```python
from build123d import *

# Parameters (mm, degrees)
BOSS_EXTRUDE1_DEPTH = 44
FILLET1_R           = 10
SKETCH5_W           = 3
SKETCH5_H           = 24
BOSS_EXTRUDE3_DEPTH = 15
FILLET4_R           = 1
CHAMFER3_SIZE       = 1


with BuildPart() as part:
    # Sketch1 → Boss-Extrude1 (new body)
    with BuildSketch(Plane.XY):
        Polygon((-20.6, 0), (20.6, 0), (20.6, 8.604532937), (-20.6, 5), align=None)
    extrude(amount=BOSS_EXTRUDE1_DEPTH)

    # Fillet1
    fillet1_edges = [part.edges().sort_by_distance(p)[0] for p in [
        (20.6, 4.302266469, 44),
        (-20.6, 2.5, 44),
        (20.6, 4.302266469, 0),
        (-20.6, 2.5, 0),
    ]]
    fillet(fillet1_edges, radius=FILLET1_R)

    # Sketch5 → Boss-Extrude3 (add)
    with BuildSketch(Plane.XZ):
        with Locations((19.1, 22)):
            Rectangle(SKETCH5_W, SKETCH5_H)
    extrude(amount=BOSS_EXTRUDE3_DEPTH)

    # Fillet4
    fillet4_edges = [part.edges().sort_by_distance(p)[0] for p in [
        (17.6, -7.5, 34),
        (17.6, -7.5, 10),
    ]]
    fillet(fillet4_edges, radius=FILLET4_R)

    # Chamfer3
    # the kernel refuses this chamfer: 1 mm, written as the material it adds along each edge
    with BuildSketch(Plane(origin=(17.6, 0, 11), x_dir=(-0.9996219169112952, 0.027495876610644465, 0), z_dir=(0, 0, 1))) as chamfer3_piece_1:
        Polygon((CHAMFER3_SIZE * 0.999621916911, CHAMFER3_SIZE * 0.0274958766106), (-CHAMFER3_SIZE * 0.0274958766106, CHAMFER3_SIZE * 0.999621916911), (0, 0), align=None)
    extrude(amount=22)
    with BuildSketch(Plane(origin=(18.6, 0, 34), x_dir=(0, 0.027495876610647806, 0.999621916911295), z_dir=(1, 0, 0))) as chamfer3_piece_2_section:
        Polygon((CHAMFER3_SIZE * 0.999621916911, CHAMFER3_SIZE * 0.0274958766106), (-CHAMFER3_SIZE * 0.0274958766106, CHAMFER3_SIZE * 0.999621916911), (0, 0), align=None)
    chamfer3_piece_2 = extrude(amount=4.571682988, mode=Mode.PRIVATE)
    chamfer3_piece_2 = chamfer3_piece_2 & Plane(origin=(10.6, -0.333892015, 34), x_dir=(1, 0, 0), z_dir=(0, 1, 0)) * Cylinder(10, 14, mode=Mode.PRIVATE)
    add(chamfer3_piece_2)
    with BuildSketch(Plane(origin=(23.171682988, 0, 10), x_dir=(0, 0.02749587661058639, -0.9996219169112968), z_dir=(-1, 0, 0))) as chamfer3_piece_3_section:
        Polygon((CHAMFER3_SIZE * 0.999621916911, CHAMFER3_SIZE * 0.0274958766106), (-CHAMFER3_SIZE * 0.0274958766106, CHAMFER3_SIZE * 0.999621916911), (0, 0), align=None)
    chamfer3_piece_3 = extrude(amount=4.571682988, mode=Mode.PRIVATE)
    chamfer3_piece_3 = chamfer3_piece_3 & Plane(origin=(10.6, -0.333892015, 10), x_dir=(1, 0, 0), z_dir=(0, 1, 0)) * Cylinder(10, 14, mode=Mode.PRIVATE)
    add(chamfer3_piece_3)
    with BuildSketch(Plane(origin=(18.6, 0, 33), x_dir=(-1, 0, 0), z_dir=(0, 0, -1))) as chamfer3_piece_4:
        Polygon((1 + CHAMFER3_SIZE, 0), (1, -CHAMFER3_SIZE), (1, 0), align=None)
    revolve(axis=Axis((18.6, 0, 33), (0, 1, 0)), revolution_arc=90)
    with BuildSketch(Plane(origin=(18.6, 0, 11), x_dir=(0, 0, -1), z_dir=(1, 0, 0))) as chamfer3_piece_5:
        Polygon((1 + CHAMFER3_SIZE, 0), (1, -CHAMFER3_SIZE), (1, 0), align=None)
    revolve(axis=Axis((18.6, 0, 11), (0, 1, 0)), revolution_arc=90)


solid = part.part
```
Check sheet for the modelled part. Datum: model origin and axes. Units: mm. A direction names the side the tool comes from. Coordinates: 2 decimals unless noted, no trailing zeros. Loops run counter-clockwise (first coordinate to the right, second up) from the corner with the lowest first, then second, coordinate; pieces in that order, holes last.
1) Sectioned sample at B-B (y = -5.25). Record the boundary of the cut face in (x, z).
2) Gauge pin test, flat ends, axial feed: pin 1 (8 mm diameter, centred on x = 16, y = 5, fed in from -Z); pin 2 (5 mm diameter, centred on x = 8.5, z = 25, fed in from +Y); pin 3 (1.6 mm diameter, centred on x = 19, y = -9, fed in from -Z). Record the tip position at first contact, or that the pin passes through.
3) Access from +Z, -Z, +X, -X, +Y, -Y to the whole of each face (thin tool, end or side, straight path). Record for faces 1 (the face through (20, -8, 10)), 2 (the face through (20, -8, 34)), 3 (the face through (17.6, -8, 22)), 4 (the face through (17.885, -8.098, 33.699)).
4) Sectioned sample at A-A (z = 18). Record the boundary of the cut face in (x, y).
5) Sectioned sample at D-D (y = 1). Record the boundary of the cut face in (x, z).
6) Sectioned sample at C-C (x = -10). Record the boundary of the cut face in (y, z).
7) Material ranges on probe 1 along X at (y, z) = (-11.5, 22); probe 2 along Y at (x, z) = (14, 33.5); probe 3 along Y at (x, z) = (13, 29), recorded low to high.
Check sheet entries:
1. outline: (17.6, 11) arc R1 ccw to (18.6, 10) - (20.6, 10) - (20.6, 34) - (18.6, 34) arc R1 ccw to (17.6, 33) - close
2. pin 1: stops at z = 0.1
2. pin 2: stops at y = 7.76
2. pin 3: stops at z = 10
3. face 1: -Z, +X, -X, -Y
3. face 2: +Z, +X, -X, -Y
3. face 3: +Z, -Z, -X, -Y
3. face 4: +Z, -X, -Y
4. outline: (-20.6, 0) - (16.6, 0) - (17.6, -1) - (17.6, -15) - (20.6, -15) - (20.6, 8.6) - (-20.6, 5) - close
5. outline: (-20.6, 10) arc R10 ccw to (-10.6, 0) - (10.6, 0) arc R10 ccw to (20.6, 10) - (20.6, 34) arc R10 ccw to (10.6, 44) - (-10.6, 44) arc R10 ccw to (-20.6, 34) - close
6. outline: (0, 0) - (5.93, 0) - (5.93, 44) - (0, 44) - close
7. probe 1: x = 17.6 to 20.6
7. probe 2: y = 0 to 8.03
7. probe 3: y = 0 to 7.94
